Can you work these out from the drawing? Everything is in mm from the part's minimum corner. A direction names the side the tool comes from. Coordinates: 2 decimals unless noted, no trailing zeros. Loops run counter-clockwise (first coordinate to the right, second up) from the corner with the lowest first, then second, coordinate; pieces in that order, holes last. Notation, with made-up numbers: (-22.75, 2) -> (36.25, 2) arc R15 cw to (36.25, 25) -> close; hole circle Ø10 at (73, 29). An arc over 180 degrees is marked (long way). Put each result on its own line as item: value. Start each with the question number.
Item 1: If we section it at C-C on y = 19.05: Please give me the cut outline in (x, z).
Item 2: If we section it at B-B on z = 2.25: Please give me the cut outline in (x, y), plus the area to 3 significant figures.
Item 3: Please list where these lines run through material, in increasing order: L1, parallel to Y at x = 20, z = 2.7; L2, parallel to X at y = 12, z = 1.95; L3, parallel to X at y = 19, z = 2.1 (1 decimal). Write a range as from..to.
Item 4: If we section it at A-A on x = 18.5: Please give me the cut outline in (y, z).
Item 5: If we section it at D-D on x = 36: Please give me the cut outline in (y, z).
Item 6: For the marked faces 1, 2 and 3, which set-ups out of +Z, -Z, +X, -X, +Y, -Y let a thin tool reach every point of the face, with its end or its side?
Item 7: Will these pins go through, and if not, where does the flat tip stop? P1, Ø1.5, axis at y = 27.5, z = 2, coming from the +X side; P2, Ø2.5, axis at x = 36.51, y = 19.05, coming from the +Z side; P3, Ø0.9, axis at y = 3.5, z = 1, coming from the -X side; P4, Ø1.5, axis at x = 36.5, z = 2, coming from the -Y side.
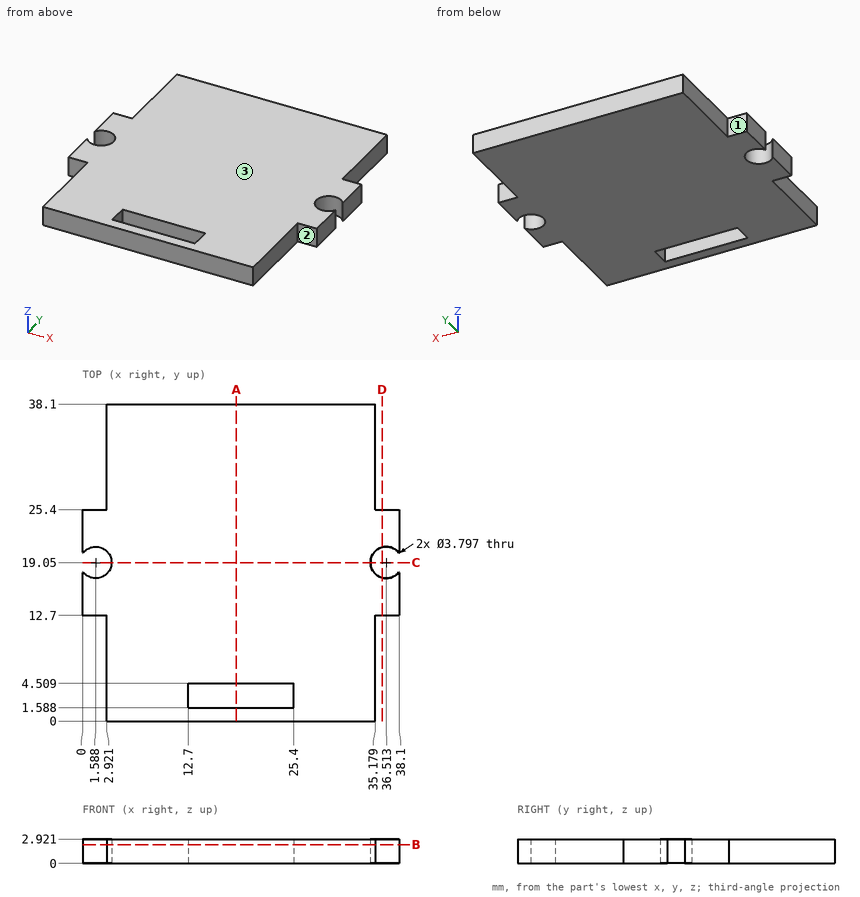
Solutions:
1. outline: (3.49, 0) -> (34.61, 0) -> (34.61, 2.92) -> (3.49, 2.92) -> close
2. outline: (0, 12.7) -> (2.92, 12.7) -> (2.92, 0) -> (35.18, 0) -> (35.18, 12.7) -> (38.1, 12.7) -> (38.1, 18.01) arc R1.9 cw (long way) to (38.1, 20.09) -> (38.1, 25.4) -> (35.18, 25.4) -> (35.18, 38.1) -> (2.92, 38.1) -> (2.92, 25.4) -> (0, 25.4) -> (0, 20.09) arc R1.9 cw (long way) to (0, 18.01) -> close; hole (12.7, 1.59) -> (25.4, 1.59) -> (25.4, 4.51) -> (12.7, 4.51) -> close
2. area: 1,240 mm^2
3. L1: 0..1.59, 4.51..38.1
3. L2: 2.92..35.18
3. L3: 3.5..34.6
4. outline: (0, 0) -> (1.59, 0) -> (1.59, 2.92) -> (0, 2.92) -> close; (4.51, 0) -> (38.1, 0) -> (38.1, 2.92) -> (4.51, 2.92) -> close
5. outline: (12.7, 0) -> (17.22, 0) -> (17.22, 2.92) -> (12.7, 2.92) -> close; (20.88, 0) -> (25.4, 0) -> (25.4, 2.92) -> (20.88, 2.92) -> close
6. face 1: +Z, -Z, -X, +Y
6. face 2: +Z, -Z, +X, -Y
6. face 3: +Z, +X, -X, +Y, -Y
7. P1: x = 35.18
7. P2: through
7. P3: x = 2.92
7. P4: y = 12.7
